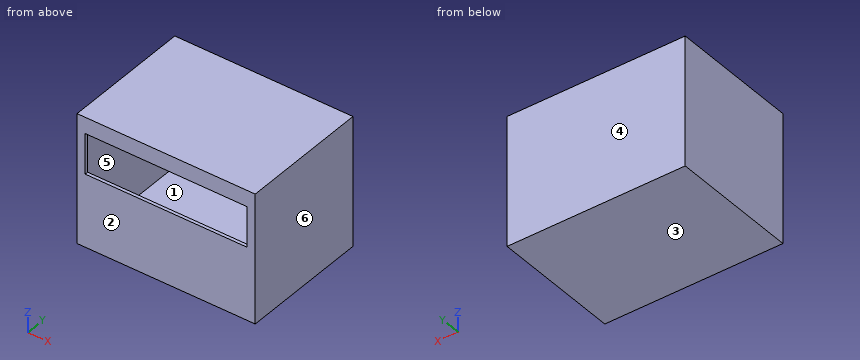
```python
from build123d import *

# Parameters (mm, degrees)
F0_W     = 139.7
F0_H     = 101.6
F1_DEPTH = 101.6
F2_T     = -2.54
F3_W     = 127
F3_H     = 31.75
F4_DEPTH = 25.4


with BuildPart() as f1:
    # F0 (on Front) → F1 (new body)
    with BuildSketch(Plane.XZ):
        with Locations((69.85, 50.8)):
            Rectangle(F0_W, F0_H)
    extrude(amount=F1_DEPTH)

    # F2 (hollow: no face is removed)
    offset(amount=F2_T, mode=Mode.SUBTRACT)

    # F3 (on face) → F4 (cut)
    with BuildSketch(Plane.XZ.offset(101.6)):
        with Locations((69.85, 73.025)):
            Rectangle(F3_W, F3_H)
    extrude(amount=-F4_DEPTH, mode=Mode.SUBTRACT)


solid = f1.part
```
The model under review builds one solid part; all positions refer to its coordinate system, in mm. Face numbers are marked on the shaded views. A direction names the side the tool comes from. Give positions to 0.01 mm unless a question says otherwise; leave off trailing zeros. Write each loop counter-clockwise with the first axis right and the second up, starting at its lowest first coordinate (ties: lowest second). Pieces come first, ordered by that corner, then holes. Notation, with made-up numbers: (12, 81) -> (67, 81) arc R28 ccw to (67, 104) -> close; hole circle Ø8 at (-35, -36). An arc over 180 degrees is marked (long way). Put each result on its own line as item: value.
(1) We need section B-B, the plane x = 98.5. Give the boundary of the cut face in (y, z).
Results are:
outline: (-101.6, 0) -> (0, 0) -> (0, 101.6) -> (-101.6, 101.6) -> (-101.6, 88.9) -> (-99.06, 88.9) -> (-99.06, 99.06) -> (-2.54, 99.06) -> (-2.54, 2.54) -> (-99.06, 2.54) -> (-99.06, 57.15) -> (-101.6, 57.15) -> close
(2) We need section A-A, the plane z = 53. Give the boundary of the cut face in (x, y), and give its area (3 significant figures).
Results are:
outline: (0, -101.6) -> (139.7, -101.6) -> (139.7, 0) -> (0, 0) -> close; hole (2.54, -99.06) -> (137.16, -99.06) -> (137.16, -2.54) -> (2.54, -2.54) -> close
area: 1,200 mm²
(3) The part is to be moulded in two halves that separate along Y. For the marked faces 1, 2, 3 and 4, say which applies: pulls with the +Y half, pulls with the -Y half, needs draft (parallel to the pull), parting line crosses it, or undercut.
Results are:
face 1: undercut
face 2: pulls with the -Y half
face 3: needs draft
face 4: pulls with the +Y half
(4) To check wall thickness, follow probe 1 along X at (y, z) = (-83, 12); probe 2 along Z at (x, y) = (23, -34.5); probe 3 along Y at (x, z) = (10, 42.5). State the ranges of each line that lie inside material, in increasing order. Write a range as from..to.
Results are:
probe 1: 0..2.54, 137.16..139.7
probe 2: 0..2.54, 99.06..101.6
probe 3: -101.6..-99.06, -2.54..0
(5) We need section C-C, the plane y = -55. Give the boundary of the cut face in (x, z).
Results are:
outline: (0, 0) -> (139.7, 0) -> (139.7, 101.6) -> (0, 101.6) -> close; hole (2.54, 2.54) -> (137.16, 2.54) -> (137.16, 99.06) -> (2.54, 99.06) -> close
(6) We need section D-D, the plane z = 71. Give the boundary of the cut face in (x, y), and give its area (3 significant figures).
Results are:
outline: (0, -101.6) -> (6.35, -101.6) -> (6.35, -99.06) -> (2.54, -99.06) -> (2.54, -2.54) -> (137.16, -2.54) -> (137.16, -99.06) -> (133.35, -99.06) -> (133.35, -101.6) -> (139.7, -101.6) -> (139.7, 0) -> (0, 0) -> close
area: 877 mm²
(7) Tool access review of the marked faces 5 and 6: name each direction out of +Z, -Z, +X, -X, +Y, -Y from which nothing blocks a thin tool from reaching the whole face with its end or side.
Results are:
face 5: none
face 6: +Z, -Z, +X, +Y, -Y
